Input: part model. Units: mm. Frame: model coordinates. Give positions to 0.01 mm unless a question says otherwise; leave off trailing zeros. Write each loop counter-clockwise with the first axis right and the second up, starting at its lowest first coordinate (ties: lowest second). Pieces come first, ordered by that corner, then holes. Notation, with made-up numbers: (84, 44) -> (109, 44) arc R21 cw to (109, 62) -> close; hole circle Ø5 at (69, 24). An arc over 180 degrees is marked (long way). Return JSON: item names as keys, results as strings. Group by question number.
Item 1: Section B-B, the plane x = 21. Return loops of the section in (y, z), then the cut area to 3 significant figures.
Item 2: Section A-A, the plane z = 3.05. Return loops of the section in (x, y).
Item 3: Pin query (flat end, axial travel): P1, Ø2, axis at y = 2.5, z = 3.5, coming from the -X side; P2, Ø1.5, axis at y = 28.5, z = 1.5, coming from the -X side; P3, Ø2, axis at x = 20.5, z = 3.5, coming from the +Y side; P4, Ø5, axis at x = 27, y = 16, coming from the -Z side. Return the tip coordinate at first contact, or that it passes through.
Item 4: Section C-C, the plane y = 32. Return loops of the section in (x, z).
Item 5: Mould query, pull axis Y, two halves, no side actions, for faces 1 (the face through (25.62, 27.82, 2.46)), 2 (the face through (42.59, 28.136, 2.535)), 3 (the face through (14.895, 5.286, 2.465)), 4 (the face through (36.573, 25.063, 2.535)). Classes: released by +Y, released by -Y, zero draft, split by the parting line, or undercut.
Item 6: Line query: line 1 (Y direction, x = 36.5, z = 2.6); line 2 (Y direction, x = 36, z = 1.5); line 3 (X direction, y = 20, z = 1.45). Output: solid intervals per line, ascending. Write a range as [from, to].
from build123d import *

# Parameters (mm, degrees)
BOSS_EXTRUDE1_DEPTH = 5
SKETCH4_R           = 1.5
CUT_EXTRUDE1_DEPTH  = 7


with BuildPart() as part:
    # Sketch3 → Boss-Extrude1 (new body)
    with BuildSketch(Plane.XY):
        with BuildLine():
            Line((0, 0), (9.528804476, 16.807257883))
            ThreePointArc((9.528804476, 16.807257883), (11.101707988, 18.890718774), (13.160255471, 20.496090072))
            Line((13.160255471, 20.496090072), (38.436867059, 35.354929207))
            ThreePointArc((38.436867059, 35.354929207), (47.786303491, 32.928139434), (45.359513719, 23.578703003))
            Line((45.359513719, 23.578703003), (16.927471829, 6.864946286))
            ThreePointArc((16.927471829, 6.864946286), (14.868924346, 5.259574989), (13.296020834, 3.176114098))
            Line((13.296020834, 3.176114098), (8.699180072, -4.931963714))
            ThreePointArc((8.699180072, -4.931963714), (1.838948591, -6.894344126), (0, 0))
        make_face()
    extrude(amount=BOSS_EXTRUDE1_DEPTH)

    # Sketch4 → Cut-Extrude1 (cut)
    with BuildSketch(Plane.XY.offset(5)):
        with Locations((41.898190389, 29.466816105)):
            Circle(SKETCH4_R)
        with Locations((36.898190389, 26.527569465)):
            Circle(SKETCH4_R)
    extrude(amount=-CUT_EXTRUDE1_DEPTH, mode=Mode.SUBTRACT)


solid = part.part
Answer below:
{
 "1": {"outline": "(9.26, 0) -> (25.1, 0) -> (25.1, 5) -> (9.26, 5) -> close", "area": "79.2 mm2"},
 "2": {"outline": "(0, 0) arc R5 ccw (long way) to (8.7, -4.93) -> (13.3, 3.18) arc R10 cw to (16.93, 6.86) -> (45.36, 23.58) arc R6.83 ccw to (38.44, 35.35) -> (13.16, 20.5) arc R10 ccw to (9.53, 16.81) -> close; hole circle Ø3 at (36.9, 26.53); hole circle Ø3 at (41.9, 29.47)"},
 "3": {"P1": "stops at x = 0.85", "P2": "stops at x = 25.5", "P3": "stops at y = 25.4", "P4": "stops at z = 0"},
 "4": {"outline": "(32.73, 0) -> (48.24, 0) -> (48.24, 5) -> (32.73, 5) -> close"},
 "5": {"face 1": "released by +Y", "face 2": "undercut", "face 3": "released by -Y", "face 4": "undercut"},
 "6": {"line 1": "y = [18.37, 25.08], [27.97, 34.22]", "line 2": "y = [18.08, 25.33], [27.73, 33.92]", "line 3": "x = [12.4, 39.27]"}
}
